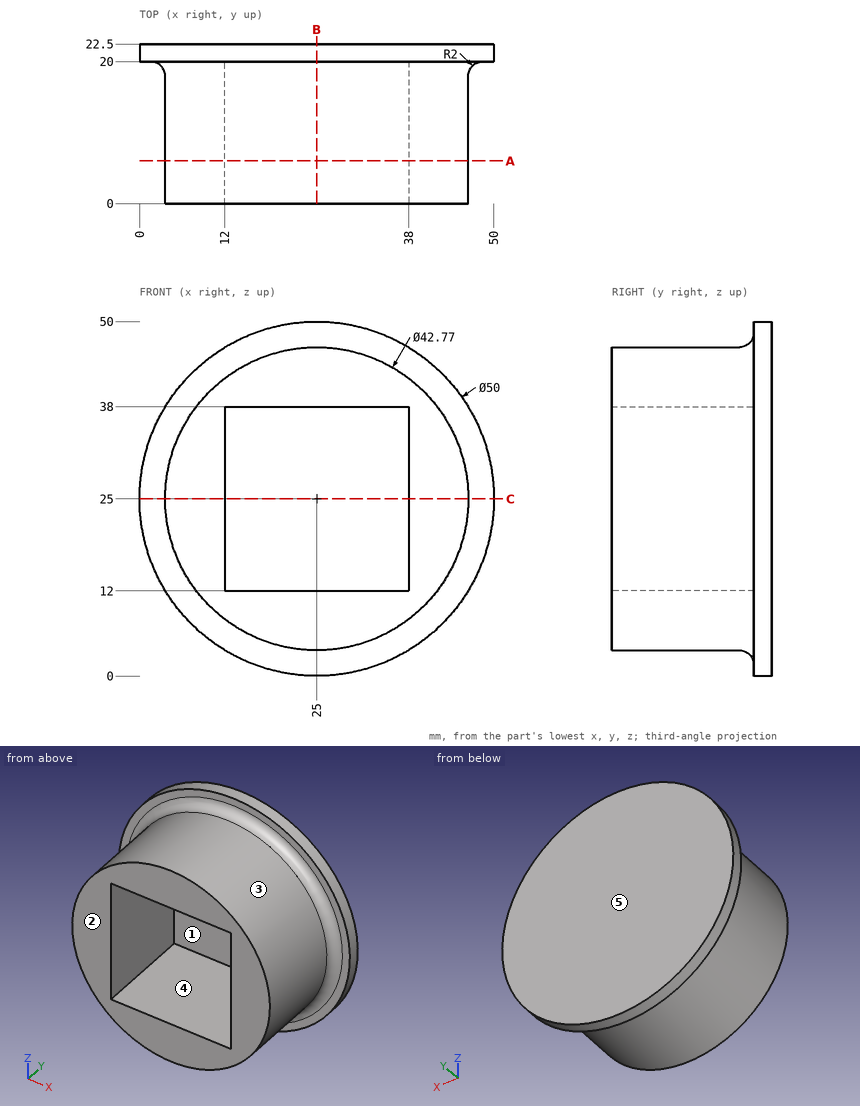
Job drawing, mm, ordinate dimensions from the low corner. One solid piece. A direction names the side the tool comes from. Give positions to 0.01 mm unless a question says otherwise; leave off trailing zeros. Write each loop counter-clockwise with the first axis right and the second up, starting at its lowest first coordinate (ties: lowest second). Pieces come first, ordered by that corner, then holes. Notation, with made-up numbers: (-17, 61.25) -> (9, 61.25) arc R12 ccw to (9, 67.25) -> close; hole circle Ø4 at (17.5, -0.75). An arc over 180 degrees is marked (long way). Return JSON: item names as keys, results as strings.
Item 1: Band-saw the part on C-C (z = 25). List the corners of the cut face in (x, y) (1 decimal), then the cut area to 3 significant figures.
Answer below:
{"outline": "(0, 20) -> (1.6, 20) arc R2 cw to (3.6, 18) -> (3.6, 0) -> (12, 0) -> (12, 20) -> (38, 20) -> (38, 0) -> (46.4, 0) -> (46.4, 18) arc R2 cw to (48.4, 20) -> (50, 20) -> (50, 22.5) -> (0, 22.5) -> close", "area": "462 mm2"}
Item 2: Two-plate mould, pull along Z, no slides. Class the marked faces 3, 4 and 5: +Z half, -Z half, draft (parallel to the pull), parting line (faces both ways), or undercut.
Answer below:
{"face 3": "parting line", "face 4": "undercut", "face 5": "draft"}
Item 3: Tool access for the marked faces 1 and 2: list every direction of +Z, -Z, +X, -X, +Y, -Y with a clear straight run to the whole face (end or side of a thin tool).
Answer below:
{"face 1": "-Y", "face 2": "+Z, -Z, +X, -X, -Y"}
Item 4: Band-saw the part on A-A (y = 6). List the corners of the cut face in (x, z) (1 decimal).
Answer below:
{"outline": "circle Ø42.8 at (25, 25); hole (12, 12) -> (38, 12) -> (38, 38) -> (12, 38) -> close"}
Item 5: Drop flat-ended pins along their axis: pin 1 (6 mm diameter, centred on x = 20, y = 15, fed in from -Z); pin 2 (12 mm diameter, centred on x = 16, y = 14.5, fed in from +Z); pin 3 (5 mm diameter, centred on y = 5, z = 18.5, fed in from -X). Give the stop position or say it passes through.
Answer below:
{"pin 1": "stops at z = 3.71", "pin 2": "stops at z = 49.11", "pin 3": "stops at x = 3.99"}
Item 6: Drill centre lines: probe 1 along Y at (x, z) = (35, 13); probe 2 along X at (y, z) = (2, 18.5); probe 3 along X at (y, z) = (12.25, 33). Where is each one in solid material? Low to high.
Answer below:
{"probe 1": "y = 20 to 22.5", "probe 2": "x = 4.63 to 12, 38 to 45.37", "probe 3": "x = 5.17 to 12, 38 to 44.83"}
Item 7: Band-saw the part on B-B (x = 25). List the corners of the cut face in (y, z) (1 decimal), then the cut area to 3 significant figures.
Answer below:
{"outline": "(0, 3.6) -> (18, 3.6) arc R2 cw to (20, 1.6) -> (20, 0) -> (22.5, 0) -> (22.5, 50) -> (20, 50) -> (20, 48.4) arc R2 cw to (18, 46.4) -> (0, 46.4) -> (0, 38) -> (20, 38) -> (20, 12) -> (0, 12) -> close", "area": "462 mm2"}
